```python
from build123d import *

# Parameters (mm, degrees)
RESSALTO_EXTRUS_O1_DEPTH = 17
ESBO_O2_R                = 2.6
CORTE_EXTRUS_O1_DEPTH    = 20
CHANFRO1_SIZE            = 8
CHANFRO1_SIZE2           = 5
ESBO_O3_R                = 1.7
CORTE_EXTRUS_O2_DEPTH    = 21
CORTE_EXTRUS_O3_START    = -3
CORTE_EXTRUS_O3_DEPTH    = 2.5


with BuildPart() as part:
    # Esboço1 → Ressalto-extrusão1 (new body)
    with BuildSketch(Plane.XY):
        Polygon((0, 0), (15, 0), (15, 12), (23, 12), (23, 20), (15, 20), (10, 15), (10, 5), (0, 5), align=None)
    extrude(amount=-RESSALTO_EXTRUS_O1_DEPTH)

    # Esboço2 → Corte-extrusão1 (cut)
    with BuildSketch(Plane(origin=(0, 5, 0), x_dir=(1, 0, 0), z_dir=(0, 1, 0))):
        with Locations((5, 10)):
            Circle(ESBO_O2_R)
    extrude(amount=-CORTE_EXTRUS_O1_DEPTH, mode=Mode.SUBTRACT)

    # Chanfro1
    chanfro1_edges = [part.edges().sort_by_distance(p)[0] for p in [
        (23, 16, -17),
    ]]
    chanfro1_side = [part.faces().sort_by_distance(p)[0] for p in [
        (12.755169562, 9.52770885, -17),
    ]]
    chamfer(chanfro1_edges, length=CHANFRO1_SIZE, length2=CHANFRO1_SIZE2, reference=chanfro1_side[0])

    # Esboço3 → Corte-extrusão2 (cut, through all)
    with BuildSketch(Plane(origin=(0, 20, 0), x_dir=(1, 0, 0), z_dir=(0, 1, 0))):
        with Locations((20, 6)):
            Circle(ESBO_O3_R)
    extrude(amount=-CORTE_EXTRUS_O2_DEPTH, mode=Mode.SUBTRACT)

    # Esboço4 → Corte-extrusão3 (cut)
    with BuildSketch(Plane(origin=(0, 20, 0), x_dir=(1, 0, 0), z_dir=(0, 1, 0)).offset(CORTE_EXTRUS_O3_START)):
        Polygon((23, 8.875), (18.340117976, 8.875), (16.680235952, 6), (18.340117976, 3.125), (23, 3.125), align=None)
    extrude(amount=-CORTE_EXTRUS_O3_DEPTH, mode=Mode.SUBTRACT)


solid = part.part
```
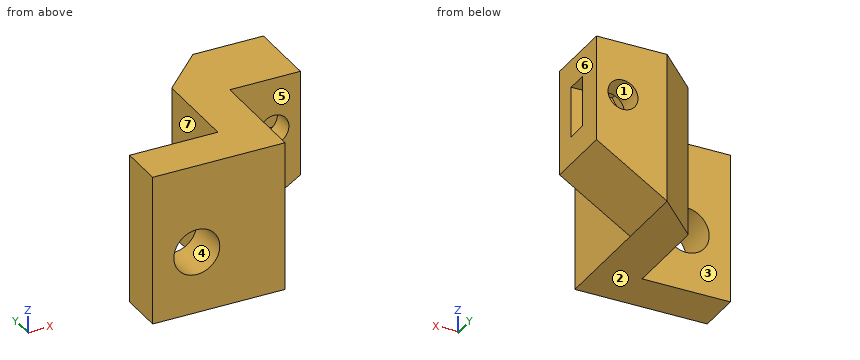
The listing builds one solid part. Answer for the finished solid, in the listing's coordinates (mm). Face numbers are marked on the shaded views. A direction names the side the tool comes from. Coordinates: 2 decimals unless noted, no trailing zeros. Loops run counter-clockwise (first coordinate to the right, second up) from the corner with the lowest first, then second, coordinate; pieces in that order, holes last. Notation, with made-up numbers: (55.5, 46) -> (87.5, 46) arc R6 ccw to (87.5, 55) -> close; hole circle Ø10 at (84, 86). An arc over 180 degrees is marked (long way). Use one line per item in the form item = value. Start each with the question number.
Item 1: The part is cut by section A-A on x = 5. Determine the outline of the cut face in (y, z).
Item 2: A tool of negligible diameter and unlimited length cuts with its end or side. For the marked faces 5, 6 and 7, from which of +Z, -Z, +X, -X, +Y, -Y can it reach the whole face along a straight path? Write none if from no direction.
Item 3: The part is cut by section B-B on z = -10. Determine the outline of the cut face in (x, y), then the cut area to 4 significant figures.
Item 4: The part is cut by section C-C on y = 13.25. Determine the outline of the cut face in (x, z), then the cut area to 3 significant figures.
Item 5: The part is cut by section D-D on z = -13.75. Determine the outline of the cut face in (x, y), then the cut area to 3 significant figures.
Item 6: Consider L1, parallel to X at y = 1.2, z = -10; L2, parallel to X at y = 12.7, z = -6; L3, parallel to Z at x = 5, y = 2.55. Determine where each line is inside the solid, lowest interval first. Write a range as [from, to].
Item 7: Flat-ended cylindrical pins translate along their axes: pin 1 Ø6.5 at (x, z) = (18.5, -5) entering from -Y; pin 2 Ø10 at (y, z) = (13.5, -2) entering from -X; pin 3 Ø0.8 at (x, y) = (20.5, 15.5) entering from -Z; pin 4 Ø2 at (x, y) = (20, 15.5) entering from +Z. Find the tip coordinate at first contact, or state that the pin passes through.
Item 8: The mould has two halves that part along Z. Classify the marked faces 1, 2, 3 and 4: released by +Z, released by -Z, zero draft, split by the parting line, or undercut.
Answer key:
q1.outline = (0, -17) -> (5, -17) -> (5, -12.6) -> (0, -12.6) -> close; (0, -7.4) -> (5, -7.4) -> (5, 0) -> (0, 0) -> close
q2.face_5 = +Z, -Z, +X, -Y
q2.face_6 = +Z, -Z, +X, +Y, -Y
q2.face_7 = +Z, -Z, -X, +Y
q3.outline = (0, 0) -> (2.4, 0) -> (2.4, 5) -> (0, 5) -> close; (7.6, 0) -> (15, 0) -> (15, 12) -> (23, 12) -> (23, 20) -> (15, 20) -> (10, 15) -> (10, 5) -> (7.6, 5) -> close
q3.area = 175.5 mm2
q4.outline = (10, -17) -> (15, -17) -> (23, -12) -> (23, 0) -> (10, 0) -> close; hole circle Ø3.4 at (20, -6)
q4.area = 192 mm2
q5.outline = (0, 0) -> (15, 0) -> (15, 12) -> (20.2, 12) -> (20.2, 20) -> (15, 20) -> (10, 15) -> (10, 5) -> (0, 5) -> close
q5.area = 179 mm2
q6.L1 = [0, 2.4], [7.6, 15]
q6.L2 = [10, 18.3], [21.7, 23]
q6.L3 = [-17, -12.6], [-7.4, 0]
q7.pin_1 = 12
q7.pin_2 = 10
q7.pin_3 = -13.81
q7.pin_4 = 0
q8.face_1 = undercut
q8.face_2 = released by -Z
q8.face_3 = zero draft
q8.face_4 = undercut
